Verification items for the finished model (mm, model axes). A direction names the side the tool comes from. Coordinates: 2 decimals unless noted, no trailing zeros. Order: outer loops, then holes, each group sorted by start corner. A loop starts at its lowest first (then second) coordinate and runs counter-clockwise, first axis right, second up. Notation, with made-up numbers: (34.25, 78) -> (72.25, 78) arc R16 cw to (72.25, 109) -> close; hole circle Ø7 at (47, 50). An arc over 180 degrees is marked (long way). Write item = value, one per line. Start each with the question number.
Autodesk Inventor part; units mm, degrees
ref_plane "YZ Plane" through (0, 0, 0) normal (1, 0, 0) x (0, 1, 0)
ref_plane "XZ Plane" through (0, 0, 0) normal (0, 1, 0) x (-1, 0, 0)
ref_plane "XY Plane" through (0, 0, 0) normal (0, 0, 1) x (1, 0, 0)
sketch "Sketch1" plane through (0, 0, 0) normal (0, 0, 1) x (1, 0, 0)
  line L0 (-75, -75) -> (75, -75)
  line L1 (75, -75) -> (75, 75)
  line L2 (75, 75) -> (-75, 75)
  line L3 (-75, 75) -> (-75, -75)
  line L4 (-75, -75) -> (75, 75) construction
  line L5 (75, -75) -> (-75, 75) construction
  arc A0 (51.4783, -11.796) -> (51.4817, 11.7813) centre (0, 0) ccw
  arc A1 (53.3699, -10.5361) -> (53.3699, 10.5361) centre (0, 0) ccw
  arc A2 (50.2551, -9.9212) -> (50.2551, 9.9212) centre (0, 0) ccw
  arc A3 (53.3699, 10.5361) -> (50.2551, 9.9212) centre (51.8125, 10.2286) ccw
  arc A4 (50.2551, -9.9212) -> (53.3699, -10.5361) centre (51.8096, -10.2434) ccw
  line L6 (0, 0) -> (120.3079, 0)
  spline S0 degree 2 poles (51.0287, -4.4801) (52.1004, -7.1283) (50.6557, -7.6159) knots 0 0 0 1 1 1
  arc A5 (54.2233, -12.4087) -> (54.2233, 12.4087) centre (0, 0) ccw
  arc A6 (48.74, -11.1539) -> (48.74, 11.1539) centre (0, 0) ccw
  arc A7 (54.2233, 12.4087) -> (48.74, 11.1539) centre (51.4817, 11.7813) ccw
  arc A8 (48.74, -11.1539) -> (54.2233, -12.4087) centre (51.4817, -11.7813) ccw
  arc A9 (53.3639, -10.5665) -> (52.4539, 14.4204) centre (0, 0) ccw
  arc A10 (50.2494, -9.9498) -> (49.3745, 13.6441) centre (0, 0) ccw
  circle A11 centre (49.4975, 49.4975) radius 5
  circle A12 centre (-49.4975, -49.4975) radius 5
  circle A13 centre (49.4975, 49.4975) radius 4
  circle A14 centre (-49.4975, -49.4975) radius 4
  point P0 (52.8125, 0)
  point P1 (28.5375, -29.3076)
  point P2 (51.5021, -11.8009)
  point P3 (51.4042, -6.894)
  point P4 (53.3699, 10.5361)
  point P5 (50.2551, 9.9212)
  dimension "d0" = 150
  dimension "d1" = 150
  dimension "d2" = 52.8125
  dimension "d6" = 102.45
  dimension "d7" = 108.8
  dimension "d8" = 4.185
  dimension "d12" = 111.25
  dimension "d13" = 100
  dimension "d21" = 10
  dimension "d22" = 10
  dimension "d23" = 8
  dimension "d24" = 8
  dimension "d39" = 70
  dimension "d40" = 70
extrude "Extrusion1" add sketch "Sketch1" against normal blind 5 contours A5 A8 A6 L6 A2 A4 A1 | L6 A1 A9 A7 A5 | L3 L2 L1 L0 | L6 A0 A3 A1 | A1 A4 A0 L6 | A3 A10 A7 A9 | L6 A2 A3 A0 | A0 A4 A2 S0 L6 | L6 A6 A7 A10 A2 | S0 A2 | A11 | A12 | A13 | A14
extrude "Extrusion2" add sketch "Sketch1" along normal blind 5 contours A5 A8 A6 L6 A2 A4 A1 | L6 A1 A9 A7 A5 | L6 A6 A7 A10 A2 | S0 A2
pattern_circular "Circular Pattern1" count 4 over 360 about axis through (0, 0, -10) along (0, 0, 1) of "Extrusion2"
extrude "Extrusion4" add sketch "Sketch1" along normal blind 9 contours A11 | A12
extrude "Extrusion5" cut sketch "Sketch1" against normal through all contours A13 | A14
fillet "Fillet1" radius 50 4 edges at (-75, 75, -2.5) (75, 75, -2.5) (75, -75, -2.5) (-75, -75, -2.5)
sketch "Sketch3" plane through (0, 0, 0) normal (0, 0, 1) x (1, 0, 0)
  circle A0 centre (0, 0) radius 35
  circle A1 centre (49.4975, 49.4975) radius 5
  line L0 (-49.4975, -49.4975) -> (49.4975, 49.4975) construction
  line L1 (49.4975, -49.4975) -> (-49.4975, 49.4975) construction
  circle A2 centre (-49.4975, 49.4975) radius 2.05
  circle A3 centre (49.4975, -49.4975) radius 2.05
  circle A4 centre (-49.4975, 49.4975) radius 5
  circle A5 centre (49.4975, -49.4975) radius 5
  dimension "d30" = 70
  dimension "d31" = 4.1
  dimension "d32" = 4.1
  dimension "d33" = 10
  dimension "d34" = 10
  dimension "d41" = 70
extrude "Extrusion6" cut sketch "Sketch3" against normal through all contours A0 | A2 | A3
extrude "Extrusion7" cut sketch "Sketch3" against normal blind 2 contours A3 | A4 | A5
equation "\"d22\" = d21"
equation "\"d24\" = d23"
properties part number "Female plug&play"
Item 1: Thickness scan on line 1 (Y direction, x = 53, z = -0.5); line 2 (Y direction, x = 7, z = 2.5); line 3 (X direction, y = -50, z = 8.5). Record the ranges inside material, lowest first.
Item 2: Mould release check, pull along X, two halves, no side actions. Record for faces 1 (the cylindrical face through (-55.625, -0.175, 2.465)), 2 (the cylindrical face through (59.964, 60.742, -2.535)), 3 (the cylindrical face through (52.94, 12.51, 2.46)): pulls with the +X half, pulls with the -X half, needs draft (parallel to the pull), parting line crosses it, or undercut.
Item 3: Section check C-C (z = 7). Record the boundary of the cut face in (x, y), then the cut area to 3 significant figures.
Item 4: Section check D-D (y = 21). Record the boundary of the cut face in (x, z), then the cut area to 3 significant figures.
Item 5: Section check A-A (y = 0). Record the boundary of the cut face in (x, z), then the cut area to 4 significant figures.
Item 6: Gauge pin test, flat ends, axial feed: P1, Ø13, axis at x = 49.5, y = 49.5, coming from the +Z side; P2, Ø5, axis at y = -41.5, z = 1, coming from the -X side; P3, Ø8, axis at y = -53.5, z = 3, coming from the -X side; P4, Ø5, axis at x = -25.5, y = -21.5, coming from the +Z side. Record the tip position at first contact, or that the pin passes through.
Item 7: Tool access check on faces 4 (the flat face through (-3.1, -50.6, 5)), 5 (the cylindrical face through (50, 0, 2)), 6 (the flat face through (3.1, 50.6, 5)). Record the directions out of +Z, -Z, +X, -X, +Y, -Y that give a thin tool (end or side, any length) a straight path to the whole face; none if there is none.
Filled sheet:
q1.line_1 = -66.42 to -53.07, -45.93 to 47.57, 51.43 to 66.42
q1.line_2 = -55.18 to -53.95, -50.74 to -49.51, 49.51 to 51.36, 53.95 to 55.18
q1.line_3 = -54.47 to -53.47, -45.53 to -44.52
q2.face_1 = pulls with the -X half
q2.face_2 = pulls with the +X half
q2.face_3 = undercut
q3.outline = circle Ø10 at (-49.5, -49.5); circle Ø10 at (49.5, 49.5); hole circle Ø8 at (-49.5, -49.5); hole circle Ø8 at (49.5, 49.5)
q3.area = 56.5 mm^2
q4.outline = (-75, -5) -> (-28, -5) -> (-28, 0) -> (-75, 0) -> close; (28, -5) -> (75, -5) -> (75, 0) -> (28, 0) -> close
q4.area = 470 mm^2
q5.outline = (-75, -5) -> (-35, -5) -> (-35, 0) -> (-50, 0) -> (-50, 5) -> (-51.23, 5) -> (-51.23, 0) -> (-54.4, 0) -> (-54.4, 5) -> (-55.63, 5) -> (-55.63, 0) -> (-75, 0) -> close; (35, -5) -> (75, -5) -> (75, 0) -> (55.63, 0) -> (55.63, 5) -> (54.4, 5) -> (54.4, 0) -> (51.23, 0) -> (51.23, 5) -> (50, 5) -> (50, 0) -> (35, 0) -> close
q5.area = 424.5 mm^2
q6.P1 = 9
q6.P2 = -72.94
q6.P3 = -67.8
q6.P4 = 0
q7.face_4 = +Z, +X, +Y, -Y
q7.face_5 = +Z
q7.face_6 = +Z, -X, +Y, -Y
